Verification items for the finished model (mm, model axes). A direction names the side the tool comes from. Round coordinates to 2 decimals unless told otherwise and drop trailing zeros. Write each loop counter-clockwise with the first axis right and the second up, starting at its lowest first coordinate (ties: lowest second). Pieces come first, ordered by that corner, then holes. Notation, with made-up numbers: M 21,-16.75 L 67,-16.75 A14 cw 67,0.25 Z; hole C 2,41 d5. An arc over 180 degrees is marked long. Use a Markdown table: item, result. Add a question column.
Autodesk Fusion 360 part; units mm, degrees
sketch "Skizze1" plane through (0, 0, 0) normal (0, 0, 1) x (1, 0, 0)
  line L0 (0, 0) -> (80, 0)
  line L1 (80, 0) -> (80, 30)
  line L2 (80, 30) -> (0, 30)
  line L3 (0, 30) -> (0, 0)
  dimension "d1" = 80
  dimension "d2" = 30
extrude "Extrusion1" add sketch "Skizze1" along normal blind 20
sketch "Skizze2" plane through (0, 0, 20) normal (0, 0, 1) x (-1, 0, 0)
  line L0 (0, -30) -> (0, 0)
  line L1 (0, 0) -> (-80, 0)
  line L2 (-80, 0) -> (-80, -30)
  line L3 (-80, -30) -> (0, -30)
  circle A0 centre (-40, -15) radius 10
  circle A1 centre (-7, -23) radius 2.5
  circle A2 centre (-7, -23) radius 4
  dimension "d5" = 20
  dimension "d6" = 40
  dimension "d7" = 15
  dimension "d8" = 5
  dimension "d9" = 8
  dimension "d10" = 7
  dimension "d11" = 7
extrude "Extrusion2" cut sketch "Skizze2" against normal blind 22 contours A0
ref_plane "Arbeitsebene1" through (40, 15, 10) normal (0, -1, 0) x (1, 0, 0)
extrude "Extrusion3" cut sketch "Skizze2" against normal blind 22 contours A1
extrude "Extrusion4" cut sketch "Skizze2" against normal blind 7 contours A2
pattern_linear "R-Anordnung1" count 2 spacing 16 along (0, -1, 0) count 2 spacing 66 along (1, 0, 0) of "Extrusion3", "Extrusion4"
sketch "Skizze3" plane through (0, 0, 0) normal (-1, 0, 0) x (0, -1, 0)
  line L0 (-30, 0) -> (0, 0)
  line L1 (0, 0) -> (0, 20)
  line L2 (0, 20) -> (-30, 20)
  line L3 (-30, 20) -> (-30, 0)
  circle A0 centre (-15, 10) radius 1.5
  dimension "d22" = 3
  dimension "d23" = 15
  dimension "d24" = 10
hole "Bohrung1" at (0, 15, 10) direction (1, 0, 0) diameter 3.332 depth 40 tip angle 118
chamfer "Fase3" distance 0.3 angle 45 1 edges at (0, 16.5533, 10.6025)
1. Cross-section at B-B on y = 15. Enter the section's corners in (x, z), plus the area to 3 significant figures.
2. Release check for a two-part mould opening along Z. For faces 3 (the cylindrical face through (5.85, 9.22, 6.59)), 4 (the cylindrical face through (15.43, 13.35, 9.78)), 5 (the flat face through (75, 9, 13)) record: +Z half, -Z half, draft (parallel to the pull), parting line (faces both ways), or undercut.
3. Access from +Z, -Z, +X, -X, +Y, -Y to the whole of each face (thin tool, end or side, straight path). Record for faces 1 (the flat face through (41, 30, 10)), 2 (the flat face through (9, 25, 13)).
4. Cross-section at A-A on x = 7. Enter the section's corners in (y, z), plus the area to 3 significant figures.
5. Scan lines: line 1 along Y through (x, z) = (7, 16); line 2 along X through (y, z) = (19.5, 16.25); line 3 along X through (y, z) = (6, 8.75). Record each from-to range of solid material in increasing order. Write a range as from..to.
6. Cross-section at D-D on x = 40. Enter the section's corners in (y, z).
7. Cross-section at C-C on z = 16.5. Enter the section's corners in (x, y), plus the area to 3 significant figures.
8. Depth check by flat-ended pin: pin 1 Ø4.5 at (x, y) = (7, 23) entering from +Z; pin 2 Ø4 at (x, y) = (5.5, 6.5) entering from +Z. Enter the tip coordinate at first touch or a pass-through.
Answer:
| question | item | result |
|---|---|---|
| 1 | outline | M 0,0 L 30,0 L 30,8.33 L 0.3,8.33 L 0,8.03 Z; M 0,11.97 L 0.3,11.67 L 30,11.67 L 30,20 L 0,20 Z; M 50,0 L 80,0 L 80,20 L 50,20 Z |
| 1 | area | 1,100 mm^2 |
| 2 | face 3 | draft |
| 2 | face 4 | undercut |
| 2 | face 5 | +Z half |
| 3 | face 1 | +Z, -Z, +X, -X, +Y |
| 3 | face 2 | +Z |
| 4 | outline | M 0,0 L 4.5,0 L 4.5,13 L 3,13 L 3,20 L 0,20 Z; M 9.5,0 L 20.5,0 L 20.5,13 L 19,13 L 19,20 L 11,20 L 11,13 L 9.5,13 Z; M 25.5,0 L 30,0 L 30,20 L 27,20 L 27,13 L 25.5,13 Z; hole C 15,10 d3.33 |
| 4 | area | 349 mm^2 |
| 5 | line 1 | y = 0..3, 11..19, 27..30 |
| 5 | line 2 | x = 0..5.06, 8.94..31.07, 48.93..71.06, 74.94..80 |
| 5 | line 3 | x = 0..4.71, 9.29..35.64, 44.36..70.71, 75.29..80 |
| 6 | outline | M 0,0 L 5,0 L 5,20 L 0,20 Z; M 25,0 L 30,0 L 30,20 L 25,20 Z |
| 7 | outline | M 0,0 L 80,0 L 80,30 L 0,30 Z; hole C 7,7 d8; hole C 7,23 d8; hole C 40,15 d20; hole C 73,7 d8; hole C 73,23 d8 |
| 7 | area | 1,880 mm^2 |
| 8 | pin 1 | passes through |
| 8 | pin 2 | stops at z = 13 |
